The model under review builds one solid part; all positions refer to its coordinate system, in mm. A direction names the side the tool comes from. Give positions to 0.01 mm unless a question says otherwise; leave off trailing zeros. Order: outer loops, then holes, each group sorted by start corner. A loop starts at its lowest first (then second) coordinate and runs counter-clockwise, first axis right, second up. Notation, with made-up numbers: (83.5, -28) - (124.5, -28) arc R21 cw to (124.5, -15) - close; hole circle Ø2 at (-29, -0.75). An arc over 180 degrees is marked (long way). Put each result on its own line as item: value.
```python
from build123d import *

# Parameters (mm, degrees)
SKETCH1_W                       = 24.3
SKETCH1_H                       = 24.3
SKETCH1_W_2                     = 14.3
SKETCH1_H_2                     = 14.3
BOSS_EXTRUDE1_DEPTH             = 4
SKETCH3_R                       = 1.5
BOSS_EXTRUDE4_DEPTH             = 4
BOSS_EXTRUDE5_DEPTH             = 4
BOSS_EXTRUDE6_REACH             = 23.355
BOSS_EXTRUDE6_DIRECTION_2_REACH = 23.355
CUT_EXTRUDE1_DEPTH              = 11
SKETCH7_W                       = 24.3
SKETCH7_H                       = 23.3
SKETCH7_W_2                     = 14.3
SKETCH7_H_2                     = 14.3
BOSS_EXTRUDE8_DEPTH             = 1
BOSS_EXTRUDE9_DEPTH             = 1.5
BOSS_EXTRUDE10_DEPTH            = 26.5
BOSS_EXTRUDE11_DEPTH            = 2
BOSS_EXTRUDE12_DEPTH            = 2
SKETCH12_R                      = 1.6
CUT_EXTRUDE2_DEPTH              = 2


with BuildPart() as part:
    # Sketch1 → Boss-Extrude1 (new body)
    with BuildSketch(Plane.XY):
        Rectangle(SKETCH1_W, SKETCH1_H)
        Rectangle(SKETCH1_W_2, SKETCH1_H_2, mode=Mode.SUBTRACT)
    extrude(amount=BOSS_EXTRUDE1_DEPTH)

    # Sketch3 → Boss-Extrude4 (add)
    with BuildSketch(Plane(origin=(0, 0, 0), x_dir=(-1, 0, 0), z_dir=(0, 0, -1))):
        with Locations(Location((8.75, 0, 0), (0, 0, 180))):
            Circle(SKETCH3_R)
        with Locations(Location((-8.75, 0, 0), (0, 0, 180))):
            Circle(SKETCH3_R)
    extrude(amount=BOSS_EXTRUDE4_DEPTH)

    # Sketch4 → Boss-Extrude5 (add)
    with BuildSketch(Plane.XY.offset(4)):
        with BuildLine():
            Line((11.248190336, -0.201777492), (11.248190336, -11.15))
            Line((11.248190336, -11.15), (14.15, -11.15))
            Line((14.15, -11.15), (14.15, 13.85))
            Line((14.15, 13.85), (-14.15, 13.85))
            Line((-14.15, 13.85), (-14.15, -11.15))
            Line((-14.15, -11.15), (-11.248190336, -11.15))
            Line((-11.248190336, -11.15), (-11.248190336, -0.201777492))
            ThreePointArc((-11.248190336, -0.201777492), (0, 11.25), (11.248190336, -0.201777492))
        make_face()
    extrude(amount=BOSS_EXTRUDE5_DEPTH)

    # Boss-Extrude6: up to this face of the body (flat: up to its plane)
    boss_extrude6_end = Plane(part.part.faces().sort_by_distance((0, 12.15, 2))[0])
    # Sketch5 → Boss-Extrude6 (add, up to the picked face)
    with BuildSketch(Plane(origin=(0, 0, 0), x_dir=(1, 0, 0), z_dir=(0, 1, 0)), mode=Mode.PRIVATE) as boss_extrude6_sk1:
        Polygon((-12.15, 0), (-14.15, -4), (-12.15, -4), align=None)
    boss_extrude6_tool1 = split(extrude(boss_extrude6_sk1.sketch, amount=BOSS_EXTRUDE6_REACH, mode=Mode.PRIVATE), bisect_by=boss_extrude6_end, keep=Keep.BOTH, mode=Mode.PRIVATE)
    # Sketch5 → Boss-Extrude6 (add, up to the picked face)
    with BuildSketch(Plane(origin=(0, 0, 0), x_dir=(1, 0, 0), z_dir=(0, 1, 0)), mode=Mode.PRIVATE) as boss_extrude6_sk2:
        Polygon((12.15, 0), (12.15, -4), (14.15, -4), align=None)
    boss_extrude6_tool2 = split(extrude(boss_extrude6_sk2.sketch, amount=BOSS_EXTRUDE6_REACH, mode=Mode.PRIVATE), bisect_by=boss_extrude6_end, keep=Keep.BOTH, mode=Mode.PRIVATE)
    add(boss_extrude6_tool1.solids().sort_by(Axis((-12.816667, 0, 2.666667), (0, 1, 0)))[0])
    add(boss_extrude6_tool2.solids().sort_by(Axis((12.816667, 0, 2.666667), (0, 1, 0)))[0])

    # Boss-Extrude6 direction 2: up to this face of the body (flat: up to its plane)
    boss_extrude6_direction_2_end = Plane(part.part.faces().sort_by_distance((12.699095168, -11.15, 6))[0])
    # Sketch5 → Boss-Extrude6 direction 2 (add, up to the picked face)
    with BuildSketch(Plane(origin=(0, 0, 0), x_dir=(1, 0, 0), z_dir=(0, 1, 0)), mode=Mode.PRIVATE) as boss_extrude6_direction_2_sk1:
        Polygon((-12.15, 0), (-14.15, -4), (-12.15, -4), align=None)
    boss_extrude6_direction_2_tool1 = split(extrude(boss_extrude6_direction_2_sk1.sketch, amount=-BOSS_EXTRUDE6_DIRECTION_2_REACH, mode=Mode.PRIVATE), bisect_by=boss_extrude6_direction_2_end, keep=Keep.BOTH, mode=Mode.PRIVATE)
    # Sketch5 → Boss-Extrude6 direction 2 (add, up to the picked face)
    with BuildSketch(Plane(origin=(0, 0, 0), x_dir=(1, 0, 0), z_dir=(0, 1, 0)), mode=Mode.PRIVATE) as boss_extrude6_direction_2_sk2:
        Polygon((12.15, 0), (12.15, -4), (14.15, -4), align=None)
    boss_extrude6_direction_2_tool2 = split(extrude(boss_extrude6_direction_2_sk2.sketch, amount=-BOSS_EXTRUDE6_DIRECTION_2_REACH, mode=Mode.PRIVATE), bisect_by=boss_extrude6_direction_2_end, keep=Keep.BOTH, mode=Mode.PRIVATE)
    add(boss_extrude6_direction_2_tool1.solids().sort_by(Axis((-12.816667, 0, 2.666667), (0, -1, 0)))[0])
    add(boss_extrude6_direction_2_tool2.solids().sort_by(Axis((12.816667, 0, 2.666667), (0, -1, 0)))[0])

    # Sketch6 → Cut-Extrude1 (cut)
    with BuildSketch(Plane.XY.offset(4)):
        Polygon((-14.15, -11.15), (-17.465023318, -11.15), (-17.465023318, -14.474968539), (16.848397365, -14.474968539), (16.848397365, -10.738940706), (14.15, -11.15), align=None)
    extrude(amount=-CUT_EXTRUDE1_DEPTH, mode=Mode.SUBTRACT)

    # Sketch7 → Boss-Extrude8 (add)
    with BuildSketch(Plane(origin=(0, 0, 0), x_dir=(-1, 0, 0), z_dir=(0, 0, -1))):
        with Locations((0, 0.5)):
            Rectangle(SKETCH7_W, SKETCH7_H)
        Rectangle(SKETCH7_W_2, SKETCH7_H_2, mode=Mode.SUBTRACT)
    extrude(amount=BOSS_EXTRUDE8_DEPTH)

    # Sketch8 → Boss-Extrude9 (add)
    with BuildSketch(Plane.XZ.offset(11.15)):
        Polygon((-14.15, 4), (-12.15, 0), (-12.15, -1), (12.15, -1), (12.15, 0), (14.15, 4), (14.15, 8), (11.248190336, 8), (11.248190336, 4), (-11.248190336, 4), (-11.248190336, 8), (-14.15, 8), align=None)
    extrude(amount=BOSS_EXTRUDE9_DEPTH)

    # Sketch9 → Boss-Extrude10 (add)
    with BuildSketch(Plane.XZ.offset(12.65)):
        Polygon((-42.15, 4), (-42.15, -11.5), (-46.15, -11.5), (-46.15, 8), (-14.15, 8), (-14.15, 4), align=None)
        Polygon((42.15, 4), (42.15, -11.5), (46.15, -11.5), (46.15, 8), (14.15, 8), (14.15, 4), align=None)
    extrude(amount=-BOSS_EXTRUDE10_DEPTH)

    # Sketch10 → Boss-Extrude11 (add)
    with BuildSketch(Plane(origin=(0, 13.85, 0), x_dir=(1, 0, 0), z_dir=(0, 1, 0))):
        Polygon((-42.15, 11.5), (-46.15, 11.5), (-46.15, -8), (46.15, -8), (46.15, 11.5), align=None)
    extrude(amount=BOSS_EXTRUDE11_DEPTH)

    # Sketch11 → Boss-Extrude12 (add)
    with BuildSketch(Plane.XZ.offset(12.65)):
        Polygon((-11.248190336, 8), (-46.15, 8), (-46.15, -11.5), (42.15, -11.5), (46.15, -11.5), (46.15, 8), (11.248190336, 8), (11.248190336, 4), (-11.248190336, 4), align=None)
    extrude(amount=BOSS_EXTRUDE12_DEPTH)

    # Sketch12 → Cut-Extrude2 (cut)
    with BuildSketch(Plane.XZ.offset(14.65)):
        with Locations((26.248190336, -7.5)):
            Circle(SKETCH12_R)
    extrude(amount=-CUT_EXTRUDE2_DEPTH, mode=Mode.SUBTRACT)


solid = part.part
```
(1) Take a section at C-C, the plane y = -5. Write out the cut boundary in (x, z), then the cut area to 3 significant figures.
The answers:
outline: (-46.15, -11.5) - (-42.15, -11.5) - (-42.15, 4) - (-14.15, 4) - (-12.15, 0) - (-12.15, -1) - (-7.15, -1) - (-7.15, 4) - (-11.25, 4) - (-11.25, 8) - (-46.15, 8) - close; (7.15, -1) - (12.15, -1) - (12.15, 0) - (14.15, 4) - (42.15, 4) - (42.15, -11.5) - (46.15, -11.5) - (46.15, 8) - (11.25, 8) - (11.25, 4) - (7.15, 4) - close
area: 461 mm^2
(2) Take a section at D-D, the plane y = 13. Write out the cut boundary in (x, z).
The answers:
outline: (-46.15, -11.5) - (-42.15, -11.5) - (-42.15, 4) - (42.15, 4) - (42.15, -11.5) - (46.15, -11.5) - (46.15, 8) - (-46.15, 8) - close
(3) The part is to be moulded in two halves that separate along Y. For faces 1 (the flat face through (0, -7.15, 2)), 2 (the flat face through (-1, 15.85, -2)), 3 (the flat face through (-1, -14.65, -2)), 4 (the cylindrical face through (-10.25, -0.07, -2.48)), say which applies: pulls with the +Y half, pulls with the -Y half, needs draft (parallel to the pull), parting line crosses it, or undercut.
The answers:
face 1: undercut
face 2: pulls with the +Y half
face 3: pulls with the -Y half
face 4: undercut
(4) Take a section at A-A, the plane x = 0. Write out the cut boundary in (y, z), then the cut area to 3 significant figures.
The answers:
outline: (-14.65, -11.5) - (-12.65, -11.5) - (-12.65, -1) - (-7.15, -1) - (-7.15, 4) - (-14.65, 4) - close; (7.15, -1) - (12.15, -1) - (12.15, 4) - (13.85, 4) - (13.85, -11.5) - (15.85, -11.5) - (15.85, 8) - (11.25, 8) - (11.25, 4) - (7.15, 4) - close
area: 133 mm^2
(5) Clearance check with flat-ended pins moving along their axes: pin 1 Ø11 at (x, y) = (1, -6) entering from +Z; pin 2 Ø4 at (x, y) = (-23, 9.5) entering from -Z; pin 3 Ø6 at (x, y) = (1, 6) entering from -Z; pin 4 Ø12 at (x, y) = (-27.5, -11) entering from -Z. State where each tip first meets the part, or that it passes through.
The answers:
pin 1: z = 4
pin 2: z = 4
pin 3: z = -1
pin 4: z = -11.5
(6) For faces 5 (the flat face through (11, 4, 8)), 6 (the flat face through (-11.248, -7, 6)), 7 (the flat face through (-4, -13, -11.5)), 8 (the flat face through (-7.15, 0, 2)), 9 (the flat face through (-9, 0, -4)), list the 3-axis set-ups (+Z, -Z, +X, -X, +Y, -Y) from which the entire face can be reached by the end or side of a thin tool; tool diameter is ignored.
The answers:
face 5: +Z, +X, -X, +Y, -Y
face 6: +Z, -Y
face 7: -Z, +X, -X, +Y, -Y
face 8: +Z, -Z
face 9: -Z
(7) Take a section at B-B, the plane z = 2.5. Write out the cut boundary in (x, y).
The answers:
outline: (-46.15, -14.65) - (46.15, -14.65) - (46.15, 15.85) - (-46.15, 15.85) - close; hole (-42.15, -12.65) - (-13.4, -12.65) - (-13.4, 12.15) - (13.4, 12.15) - (13.4, -12.65) - (42.15, -12.65) - (42.15, 13.85) - (-42.15, 13.85) - close; hole (-7.15, -7.15) - (7.15, -7.15) - (7.15, 7.15) - (-7.15, 7.15) - close
(8) Wall thickness on L1, parallel to X at y = 0.5, z = 6.25; L2, parallel to Y at x = -26, z = -0.5; L3, parallel to X at y = -5.5, z = 2.75 (3 decimals): over which ranges is each line inside the solid? List them lowest first.
The answers:
L1: -46.15 to -11.24, 11.24 to 46.15
L2: -14.65 to -12.65, 13.85 to 15.85
L3: -46.15 to -42.15, -13.525 to -7.15, 7.15 to 13.525, 42.15 to 46.15
